The listing builds one solid part. Answer for the finished solid, in the listing's coordinates (mm). Face numbers are marked on the shaded views. Coordinates: 2 decimals unless noted, no trailing zeros. Loops run counter-clockwise (first coordinate to the right, second up) from the corner with the lowest first, then second, coordinate; pieces in that order, holes last. Notation, with made-up numbers: (-31, 4) - (-17, 4) arc R31 cw to (-17, 36) - close; hole circle Ø9 at (-34, 22). An arc over 180 degrees is marked (long way). Put each result on its own line as item: value.
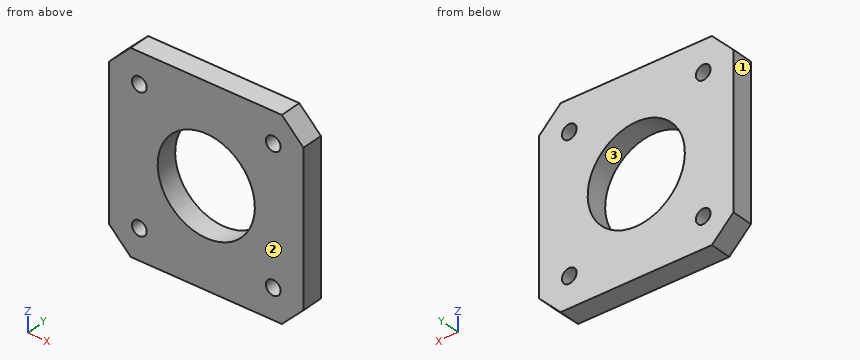
Solid Edge part; units mm, degrees
sketch "Sketch1" plane through (0, 0, 0) normal (0, -1, 0) x (1, 0, 0)
  line L0 (-22.5, -22.5) -> (22.5, -22.5)
  line L1 (22.5, -22.5) -> (22.5, 22.5)
  line L2 (22.5, 22.5) -> (-22.5, 22.5)
  line L3 (-22.5, 22.5) -> (-22.5, -22.5)
  dimension "D1" = 22.5
extrude "Protrusion1" add sketch "Sketch1" against normal blind 5
chamfer "Chamfer_1" distance 5 angle 45 4 edges at (22.5, 2.5, 22.5) (22.5, 2.5, -22.5) (-22.5, 2.5, 22.5) (-22.5, 2.5, -22.5)
hole "Hole_1" at (-15.5, 5, 15.5) direction (0, -1, 0) diameter 3.4 end up to next
hole "Hole1" at (-15.5, 5, -15.5) direction (0, -1, 0) diameter 3.4 end up to next
hole "Hole2" at (15.5, 5, -15.5) direction (0, -1, 0) diameter 3.4 end up to next
hole "Hole3" at (15.5, 5, 15.5) direction (0, -1, 0) diameter 3.4 end up to next
sketch "Sketch2" plane through (0, 5, 0) normal (0, 1, 0) x (0, 0, -1)
  circle A0 centre (0, 0) radius 11.25
extrude "Cutout1" cut sketch "Sketch2" against normal up to next
properties material "Polyethylene, low density"
1) For a pull along X with two mould halves and no side action, classify the marked faces 1, 2 and 3 as pulls with the +X half, pulls with the -X half, needs draft (parallel to the pull), parting line crosses it, or undercut.
Found:
face 1: pulls with the -X half
face 2: needs draft
face 3: undercut
2) The part is cut by section B-B (y = 0.9). Give the vertices of the cut face in (x, z).
Found:
outline: (-22.5, -17.5) - (-17.5, -22.5) - (17.5, -22.5) - (22.5, -17.5) - (22.5, 17.5) - (17.5, 22.5) - (-17.5, 22.5) - (-22.5, 17.5) - close; hole circle Ø3.4 at (-15.5, -15.5); hole circle Ø3.4 at (-15.5, 15.5); hole circle Ø22.5 at (0, 0); hole circle Ø3.4 at (15.5, -15.5); hole circle Ø3.4 at (15.5, 15.5)
3) Straight lines are drawn through the part: L1, parallel to X at y = 3.55, z = -15.5; L2, parallel to Z at x = -16, y = 4.65. For each, find the intervals that lie inside material, in ascending order. Write a range as [from, to].
Found:
L1: x = [-22.5, -17.2], [-13.8, 13.8], [17.2, 22.5]
L2: z = [-22.5, -17.12], [-13.88, 13.88], [17.12, 22.5]
4) The part is cut by section D-D (z = 15.5). Give the vertices of the cut face in (x, y), and give its area (3 significant figures).
Found:
outline: (-22.5, 0) - (-17.2, 0) - (-17.2, 5) - (-22.5, 5) - close; (-13.8, 0) - (13.8, 0) - (13.8, 5) - (-13.8, 5) - close; (17.2, 0) - (22.5, 0) - (22.5, 5) - (17.2, 5) - close
area: 191 mm^2
5) The part is cut by section C-C (x = 0). Give the vertices of the cut face in (y, z), and give its area (4 significant figures).
Found:
outline: (0, -22.5) - (5, -22.5) - (5, -11.25) - (0, -11.25) - close; (0, 11.25) - (5, 11.25) - (5, 22.5) - (0, 22.5) - close
area: 112.5 mm^2
6) The part is cut by section A-A (z = -9). Give the vertices of the cut face in (x, y).
Found:
outline: (-22.5, 0) - (-6.75, 0) - (-6.75, 5) - (-22.5, 5) - close; (6.75, 0) - (22.5, 0) - (22.5, 5) - (6.75, 5) - close
